from build123d import *

# Parameters (mm, degrees)
ESQUISSE2_W         = 216
ESQUISSE2_H         = 166
ESQUISSE2_W_2       = 210
ESQUISSE2_H_2       = 160
BOSS_EXTRU_1_DEPTH  = 25
ESQUISSE4_W         = 210
ESQUISSE4_H         = 160
BOSS_EXTRU_3_DEPTH  = 3
CONG_2_R            = 2
CONG_3_R            = 2
CONG_4_R            = 2
CONG_5_R            = 2
ESQUISSE19_R        = 1
BOSS_EXTRU_8_DEPTH  = 3
ESQUISSE18_R        = 1
BOSS_EXTRU_9_DEPTH  = 3
ESQUISSE17_R        = 1
BOSS_EXTRU_10_DEPTH = 3
ESQUISSE14_R        = 1
BOSS_EXTRU_11_DEPTH = 3


with BuildPart() as part:
    # Esquisse2 → Boss.-Extru.1 (new body)
    with BuildSketch(Plane(origin=(0, 0, 0), x_dir=(1, 0, 0), z_dir=(0, 1, 0))):
        with Locations((51.031114613, -20.511820558)):
            Rectangle(ESQUISSE2_W, ESQUISSE2_H)
        with Locations((51.031114613, -20.511820558)):
            Rectangle(ESQUISSE2_W_2, ESQUISSE2_H_2, mode=Mode.SUBTRACT)
    extrude(amount=BOSS_EXTRU_1_DEPTH)

    # Esquisse4 → Boss.-Extru.3 (add)
    with BuildSketch(Plane(origin=(0, 0, 0), x_dir=(1, 0, 0), z_dir=(0, 1, 0))):
        with Locations((51.031114613, -20.511820558)):
            Rectangle(ESQUISSE4_W, ESQUISSE4_H)
    extrude(amount=BOSS_EXTRU_3_DEPTH)

    # Congé2
    cong_2_edges = [part.edges().sort_by_distance(p)[0] for p in [
        (159.031114613, 12.5, -62.488179442),
    ]]
    fillet(cong_2_edges, radius=CONG_2_R)

    # Congé3
    cong_3_edges = [part.edges().sort_by_distance(p)[0] for p in [
        (159.031114613, 12.5, 103.511820558),
    ]]
    fillet(cong_3_edges, radius=CONG_3_R)

    # Congé4
    cong_4_edges = [part.edges().sort_by_distance(p)[0] for p in [
        (-56.968885387, 12.5, 103.511820558),
    ]]
    fillet(cong_4_edges, radius=CONG_4_R)

    # Congé5
    cong_5_edges = [part.edges().sort_by_distance(p)[0] for p in [
        (-56.968885387, 12.5, -62.488179442),
    ]]
    fillet(cong_5_edges, radius=CONG_5_R)

    # Esquisse19 → Boss.-Extru.8 (add)
    with BuildSketch(Plane(origin=(0, 25, 0), x_dir=(1, 0, 0), z_dir=(0, 1, 0))):
        with Locations((-55.168885387, 60.688179442)):
            Circle(ESQUISSE19_R)
    extrude(amount=BOSS_EXTRU_8_DEPTH)

    # Esquisse18 → Boss.-Extru.9 (add)
    with BuildSketch(Plane(origin=(0, 25, 0), x_dir=(1, 0, 0), z_dir=(0, 1, 0))):
        with Locations((-55.168885387, -101.711820558)):
            Circle(ESQUISSE18_R)
    extrude(amount=BOSS_EXTRU_9_DEPTH)

    # Esquisse17 → Boss.-Extru.10 (add)
    with BuildSketch(Plane(origin=(0, 25, 0), x_dir=(1, 0, 0), z_dir=(0, 1, 0))):
        with Locations((157.231114613, -101.711820558)):
            Circle(ESQUISSE17_R)
    extrude(amount=BOSS_EXTRU_10_DEPTH)

    # Esquisse14 → Boss.-Extru.11 (add)
    with BuildSketch(Plane(origin=(0, 25, 0), x_dir=(1, 0, 0), z_dir=(0, 1, 0))):
        with Locations((157.231114613, 60.688179442)):
            Circle(ESQUISSE14_R)
    extrude(amount=BOSS_EXTRU_11_DEPTH)


solid = part.part
Verification items for the finished model (mm, model axes). A direction names the side the tool comes from. Coordinates: 2 decimals unless noted, no trailing zeros. Order: outer loops, then holes, each group sorted by start corner. A loop starts at its lowest first (then second) coordinate and runs counter-clockwise, first axis right, second up. Notation, with made-up numbers: M 38,-8 L 63,-8 A16 ccw 63,20 Z; hole C -27,44 d1. An arc over 180 degrees is marked long. One line per item, written item: value. Start each with the question number.
Item 1: Sectioned sample at C-C (x = 10). Enter the section's corners in (y, z).
Item 2: Sectioned sample at B-B (z = 91.5). Enter the section's corners in (x, y), then the cut area to 3 significant figures.
Item 3: Sectioned sample at A-A (y = 7.5). Enter the section's corners in (x, z), then the cut area to 3 significant figures.
Item 4: Access from +Z, -Z, +X, -X, +Y, -Y to the whole of each face (thin tool, end or side, straight path). Record for faces 1 (the flat face through (50, 14, -59.488)), 2 (the flat face through (50, 0, 19)).
Item 5: Mould release check, pull along Z, two halves, no side actions. Record for faces 3 (the flat face through (50, 12, -62.488)), 4 (the flat face through (50, 3, 19)), 5 (the flat face through (159.031, 12, 22)): released by +Z, released by -Z, zero draft, split by the parting line, or undercut.
Item 6: Gauge pin test, flat end, axial feed: pin 1 (5 mm diameter, centred on x = 109.5, z = 60.5, fed in from +Y). Record the tip position at first contact, or that the pin passes through.
Item 7: Scan lines: probe 1 along Z at (x, y) = (92, 9.75); probe 2 along X at (y, z) = (14.25, -4.5); probe 3 along Y at (x, z) = (149, 85.5). Record each from-to range of solid material in increasing order.
Conclusion:
1. outline: M 0,-62.49 L 25,-62.49 L 25,-59.49 L 3,-59.49 L 3,100.51 L 25,100.51 L 25,103.51 L 0,103.51 Z
2. outline: M -56.97,0 L 159.03,0 L 159.03,25 L 156.03,25 L 156.03,3 L -53.97,3 L -53.97,25 L -56.97,25 Z
2. area: 780 mm^2
3. outline: M -56.97,-60.49 A2 ccw -54.97,-62.49 L 157.03,-62.49 A2 ccw 159.03,-60.49 L 159.03,101.51 A2 ccw 157.03,103.51 L -54.97,103.51 A2 ccw -56.97,101.51 Z; hole M -53.97,-59.49 L 156.03,-59.49 L 156.03,100.51 L -53.97,100.51 Z
3. area: 2,250 mm^2
4. face 1: +Y
4. face 2: +Z, -Z, +X, -X, -Y
5. face 3: released by -Z
5. face 4: undercut
5. face 5: zero draft
6. pin 1: stops at y = 3
7. probe 1: z = -62.49 to -59.49, 100.51 to 103.51
7. probe 2: x = -56.97 to -53.97, 156.03 to 159.03
7. probe 3: y = 0 to 3
